from build123d import *

# Parameters (mm, degrees)
SKETCH1_W           = 381
SKETCH1_H           = 508
SKETCH1_W_2         = 192
SKETCH1_H_2         = 384
BOSS_EXTRUDE1_DEPTH = 13.1
SKETCH11_R          = 1.25
CUT_EXTRUDE4_DEPTH  = 10
SKETCH12_R          = 1.25
CUT_EXTRUDE5_DEPTH  = 10
SKETCH19_R          = 1.25
CUT_EXTRUDE6_DEPTH  = 10
SKETCH20_W          = 89.5
SKETCH20_H          = 508
CUT_EXTRUDE7_DEPTH  = 10
SKETCH21_W          = 202
SKETCH21_H          = 42
CUT_EXTRUDE8_DEPTH  = 10


with BuildPart() as part:
    # Sketch1 → Boss-Extrude1 (new body)
    with BuildSketch(Plane.XY):
        with Locations((190.5, 254)):
            Rectangle(SKETCH1_W, SKETCH1_H)
        with Locations((190.5, 254)):
            Rectangle(SKETCH1_W_2, SKETCH1_H_2, mode=Mode.SUBTRACT)
    extrude(amount=BOSS_EXTRUDE1_DEPTH)

    # Sketch11 → Cut-Extrude4 (cut)
    with BuildSketch(Plane.XY.offset(13.1)):
        with Locations((107.5, 456)):
            Circle(SKETCH11_R)
    extrude(amount=-CUT_EXTRUDE4_DEPTH, mode=Mode.SUBTRACT)

    # Sketch12 → Cut-Extrude5 (cut)
    with BuildSketch(Plane.XY.offset(13.1)):
        with Locations((273.5, 456)):
            Circle(SKETCH12_R)
        with Locations((107.5, 52)):
            Circle(SKETCH12_R)
        with Locations((273.5, 52)):
            Circle(SKETCH12_R)
    extrude(amount=-CUT_EXTRUDE5_DEPTH, mode=Mode.SUBTRACT)

    # Sketch19 → Cut-Extrude6 (cut)
    with BuildSketch(Plane.XY.offset(13.1)):
        with Locations((190.5, 456)):
            Circle(SKETCH19_R)
        with Locations((190.5, 52)):
            Circle(SKETCH19_R)
    extrude(amount=-CUT_EXTRUDE6_DEPTH, mode=Mode.SUBTRACT)

    # Sketch20 → Cut-Extrude7 (cut)
    with BuildSketch(Plane.XY.offset(13.1)):
        with Locations((44.75, 254)):
            Rectangle(SKETCH20_W, SKETCH20_H)
        with Locations((336.25, 254)):
            Rectangle(SKETCH20_W, SKETCH20_H)
    extrude(amount=-CUT_EXTRUDE7_DEPTH, mode=Mode.SUBTRACT)

    # Sketch21 → Cut-Extrude8 (cut)
    with BuildSketch(Plane.XY.offset(13.1)):
        with Locations((190.5, 487)):
            Rectangle(SKETCH21_W, SKETCH21_H)
        with Locations((190.5, 21)):
            Rectangle(SKETCH21_W, SKETCH21_H)
    extrude(amount=-CUT_EXTRUDE8_DEPTH, mode=Mode.SUBTRACT)


solid = part.part
Could you check a few things on this model? Use its own coordinates, in mm. A direction names the side the tool comes from. Coordinates: 2 decimals unless noted, no trailing zeros. Write each loop counter-clockwise with the first axis right and the second up, starting at its lowest first coordinate (ties: lowest second). Pieces come first, ordered by that corner, then holes. Notation, with made-up numbers: (69.5, 40) - (73.5, 40) arc R20 cw to (73.5, 49) - close; hole circle Ø10 at (82.5, -5.75). An arc over 180 degrees is marked (long way). Put each result on its own line as item: value. Start each with the question number.
Q1. I'm going to push flat-ended pins straight in: P1, Ø4, axis at x = 273.5, y = 456, coming from the -Z side; P2, Ø5, axis at x = 225.5, z = 8.5, coming from the -Y side; P3, Ø0.8, axis at x = 190, y = 456, coming from the +Z side; P4, Ø3, axis at x = 225, z = 6.5, coming from the +Y side. Where does each tip first touch, or does it pass through?
Q2. I want a section at A-A on x = 213.5. Write out the boundary of the cut face in (y, z).
Q3. I want a section at B-B on z = 9. Write out the boundary of the cut face in (x, y).
Q4. Thinking about a two-plate mould opening in Y: for faces 1 (the flat face through (94.5, 251, 6)), 2 (the flat face through (189, 466, 8)), 3 (the flat face through (61, 258, 0)), 4 (the flat face through (189, 446, 6)), which applies, pulls with the +Y half, pulls with the -Y half, needs draft (parallel to the pull), parting line crosses it, or undercut?
Q5. I want a section at D-D on x = 73.5. Write out the boundary of the cut face in (y, z).
Q6. Please list where these lines run through material, in increasing order: L1, parallel to Y at x = 273.5, z = 10; L2, parallel to X at y = 456, z = 7; L3, parallel to X at y = 211, z = 9.
Q7. I want a section at C-C on y = 269.5. Write out the boundary of the cut face in (x, z), plus the area to 3 significant figures.
Q8. Which directions (+Z, -Z, +X, -X, +Y, -Y) give clear straight access to the entire face, cutting with the end or side of a thin tool? Please do faces 5 (the flat face through (189, 42, 8)), 6 (the flat face through (286.5, 251, 6)), 7 (the flat face through (89.5, 251, 8)).
Checks:
1. P1: z = 0
1. P2: y = 42
1. P3: z = 3.1
1. P4: y = 466
2. outline: (0, 0) - (62, 0) - (62, 13.1) - (42, 13.1) - (42, 3.1) - (0, 3.1) - close; (446, 0) - (508, 0) - (508, 3.1) - (466, 3.1) - (466, 13.1) - (446, 13.1) - close
3. outline: (89.5, 42) - (291.5, 42) - (291.5, 466) - (89.5, 466) - close; hole (94.5, 62) - (286.5, 62) - (286.5, 446) - (94.5, 446) - close; hole circle Ø2.5 at (107.5, 52); hole circle Ø2.5 at (107.5, 456); hole circle Ø2.5 at (190.5, 52); hole circle Ø2.5 at (190.5, 456); hole circle Ø2.5 at (273.5, 52); hole circle Ø2.5 at (273.5, 456)
4. face 1: undercut
4. face 2: pulls with the +Y half
4. face 3: needs draft
4. face 4: undercut
5. outline: (0, 0) - (508, 0) - (508, 3.1) - (0, 3.1) - close
6. L1: 42 to 50.75, 53.25 to 62, 446 to 454.75, 457.25 to 466
6. L2: 89.5 to 106.25, 108.75 to 189.25, 191.75 to 272.25, 274.75 to 291.5
6. L3: 89.5 to 94.5, 286.5 to 291.5
7. outline: (0, 0) - (94.5, 0) - (94.5, 13.1) - (89.5, 13.1) - (89.5, 3.1) - (0, 3.1) - close; (286.5, 0) - (381, 0) - (381, 3.1) - (291.5, 3.1) - (291.5, 13.1) - (286.5, 13.1) - close
7. area: 686 mm²
8. face 5: +Z, +X, -X, -Y
8. face 6: +Z, -Z
8. face 7: +Z, -X, +Y, -Y
